Read the model definition and answer for the solid it produces. Units are mm, in the model's axes. Face numbers are marked on the shaded views. A direction names the side the tool comes from. Coordinates: 2 decimals unless noted, no trailing zeros. Loops run counter-clockwise (first coordinate to the right, second up) from the corner with the lowest first, then second, coordinate; pieces in that order, holes last. Notation, with made-up numbers: (59, 72) -> (111, 72) arc R20 ccw to (111, 105) -> close; hole circle Ø1 at (23, -21.75). An arc over 180 degrees is marked (long way). Answer as a JSON object with one key per item and string values. Group by question number.
1) Section B-B, the plane y = -0.5 is taken. Give the vertices of the cut face in (x, z), plus the area to 3 significant figures.
2) Which of the six approach directions +Z, -Z, +X, -X, +Y, -Y give full straight-line access (tool end or side, diameter ignored) to the marked faces 5 and 6?
3) Section C-C, the plane y = -6.5 is taken. Count the separate pieces of the cut face and the enclosed holes in it, plus the area to 3 significant figures.
4) Consider probe 1 along X at (y, z) = (-4, 12.25); probe 2 along Z at (x, y) = (45.5, -9.5); probe 3 along X at (y, z) = (2.5, 14.75). Determine where each line is inside the solid, lowest interval first. Write a range as [from, to].
5) Section D-D, the plane x = 41.5 is taken. Give the vertices of the cut face in (y, z), plus the area to 3 significant figures.
6) Section A-A, the plane x = 4.5 is taken. Give the vertices of the cut face in (y, z), plus the area to 3 significant figures.
7) Determine the mould class of the marked faces 1, 2, 3 and 4 for opening direction X: released by +X, released by -X, zero draft, split by the parting line, or undercut.
8) Flat-ended cylindrical pins translate along their axes: P1, Ø5, axis at x = 36.5, z = 13, coming from the +Y side; P2, Ø2, axis at x = 28, y = -6.5, coming from the -Z side. Find the tip coordinate at first contact, or state that the pin passes through.
from build123d import *

# Parameters (mm, degrees)
PRISM004_DEPTH            = 3
CYLINDER006_R             = 1.75
CYLINDER006_DEPTH         = 20
BOX006_W                  = 6
BOX006_H                  = 20
BOX006_DEPTH              = 3
FUSION004_PLACEMENT_ANGLE = 180
PRISM005_DEPTH            = 3
CYLINDER007_R             = 1.75
CYLINDER007_DEPTH         = 20
BOX007_W                  = 6
BOX007_H                  = 20
BOX007_DEPTH              = 3
FUSION005_PLACEMENT_ANGLE = 180
PRISM002_DEPTH            = 3
CYLINDER004_R             = 1.75
CYLINDER004_DEPTH         = 20
BOX003_W                  = 6
BOX003_H                  = 20
BOX003_DEPTH              = 3
FUSION001_PLACEMENT_ANGLE = 180
PRISM003_DEPTH            = 3
CYLINDER005_R             = 1.75
CYLINDER005_DEPTH         = 20
BOX005_W                  = 6
BOX005_H                  = 20
BOX005_DEPTH              = 3
FUSION002_PLACEMENT_ANGLE = 180
FUSION007_PLACEMENT_ANGLE = 180
PRISM006_DEPTH            = 3
CYLINDER008_R             = 1.75
CYLINDER008_DEPTH         = 20
BOX008_W                  = 6
BOX008_H                  = 20
BOX008_DEPTH              = 3
FUSION008_ROLL_ANGLE      = 90
FUSION008_PLACEMENT_ANGLE = 180
PRISM007_DEPTH            = 3
CYLINDER009_R             = 1.75
CYLINDER009_DEPTH         = 20
BOX009_W                  = 6
BOX009_H                  = 20
BOX009_DEPTH              = 3
FUSION009_ROLL_ANGLE      = 90
FUSION009_PLACEMENT_ANGLE = 180
CYLINDER001_R             = 1.5
CYLINDER001_DEPTH         = 10
CYLINDER_R                = 1.5
CYLINDER_DEPTH            = 10
BOX001_W                  = 46.6
BOX001_H                  = 10
BOX001_DEPTH              = 21
BOX_W                     = 49
BOX_H                     = 5
BOX_DEPTH                 = 15
BOX004_W                  = 49
BOX004_H                  = 16
BOX004_DEPTH              = 15


with BuildPart() as prisma004:
    # Prism004 → Prism004 (new body)
    with BuildSketch(Plane(origin=(34, 7.5, 3), x_dir=(0, 1, 0), z_dir=(0, 0, 1))):
        Polygon((3.25, 0), (1.625, 2.814583), (-1.625, 2.814583), (-3.25, 0), (-1.625, -2.814583), (1.625, -2.814583), align=None)
    extrude(amount=PRISM004_DEPTH)


with BuildPart() as cilindro006:
    # Cylinder006 → Cylinder006 (new body)
    with BuildSketch(Plane(origin=(34, 7.5, -1), x_dir=(1, 0, 0), z_dir=(0, 0, 1))):
        Circle(CYLINDER006_R)
    extrude(amount=CYLINDER006_DEPTH)


with BuildPart() as fusion004:
    # Box006 → Box006 (new body)
    with BuildSketch(Plane(origin=(31, 9, 3), x_dir=(1, 0, 0), z_dir=(0, 0, 1))):
        with Locations((3, 10)):
            Rectangle(BOX006_W, BOX006_H)
    extrude(amount=BOX006_DEPTH)

    # Fusion004: union Prisma004, Cilindro006
    add(prisma004.part)
    add(cilindro006.part)


with BuildPart() as fusion004_1:
    # Fusion004 placement: moved
    add(fusion004.part.moved(Location((-14, -3, 16))).rotate(Axis((-14, -3, 16), (1, 0, 0)), FUSION004_PLACEMENT_ANGLE))


with BuildPart() as prisma005:
    # Prism005 → Prism005 (new body)
    with BuildSketch(Plane(origin=(34, 7.5, 3), x_dir=(0, 1, 0), z_dir=(0, 0, 1))):
        Polygon((3.25, 0), (1.625, 2.814583), (-1.625, 2.814583), (-3.25, 0), (-1.625, -2.814583), (1.625, -2.814583), align=None)
    extrude(amount=PRISM005_DEPTH)


with BuildPart() as cilindro007:
    # Cylinder007 → Cylinder007 (new body)
    with BuildSketch(Plane(origin=(34, 7.5, -1), x_dir=(1, 0, 0), z_dir=(0, 0, 1))):
        Circle(CYLINDER007_R)
    extrude(amount=CYLINDER007_DEPTH)


with BuildPart() as fusion006:
    # Box007 → Box007 (new body)
    with BuildSketch(Plane(origin=(31, 9, 3), x_dir=(1, 0, 0), z_dir=(0, 0, 1))):
        with Locations((3, 10)):
            Rectangle(BOX007_W, BOX007_H)
    extrude(amount=BOX007_DEPTH)

    # Fusion005: union Prisma005, Cilindro007
    add(prisma005.part)
    add(cilindro007.part)


with BuildPart() as fusion006_1:
    # Fusion005 placement: moved
    add(fusion006.part.moved(Location((2, -3, 16))).rotate(Axis((2, -3, 16), (1, 0, 0)), FUSION005_PLACEMENT_ANGLE))

    # Fusion006: union Fusion004
    add(fusion004_1.part)


with BuildPart() as prisma002:
    # Prism002 → Prism002 (new body)
    with BuildSketch(Plane(origin=(34, 7.5, 3), x_dir=(0, 1, 0), z_dir=(0, 0, 1))):
        Polygon((3.25, 0), (1.625, 2.814583), (-1.625, 2.814583), (-3.25, 0), (-1.625, -2.814583), (1.625, -2.814583), align=None)
    extrude(amount=PRISM002_DEPTH)


with BuildPart() as cilindro004:
    # Cylinder004 → Cylinder004 (new body)
    with BuildSketch(Plane(origin=(34, 7.5, -1), x_dir=(1, 0, 0), z_dir=(0, 0, 1))):
        Circle(CYLINDER004_R)
    extrude(amount=CYLINDER004_DEPTH)


with BuildPart() as fusion001:
    # Box003 → Box003 (new body)
    with BuildSketch(Plane(origin=(31, 9, 3), x_dir=(1, 0, 0), z_dir=(0, 0, 1))):
        with Locations((3, 10)):
            Rectangle(BOX003_W, BOX003_H)
    extrude(amount=BOX003_DEPTH)

    # Fusion001: union Prisma002, Cilindro004
    add(prisma002.part)
    add(cilindro004.part)


with BuildPart() as fusion001_1:
    # Fusion001 placement: moved
    add(fusion001.part.moved(Location((47, -3, 0))).rotate(Axis((47, -3, 0), (0, 0, 1)), FUSION001_PLACEMENT_ANGLE))


with BuildPart() as prisma003:
    # Prism003 → Prism003 (new body)
    with BuildSketch(Plane(origin=(34, 7.5, 3), x_dir=(0, 1, 0), z_dir=(0, 0, 1))):
        Polygon((3.25, 0), (1.625, 2.814583), (-1.625, 2.814583), (-3.25, 0), (-1.625, -2.814583), (1.625, -2.814583), align=None)
    extrude(amount=PRISM003_DEPTH)


with BuildPart() as cilindro005:
    # Cylinder005 → Cylinder005 (new body)
    with BuildSketch(Plane(origin=(34, 7.5, -1), x_dir=(1, 0, 0), z_dir=(0, 0, 1))):
        Circle(CYLINDER005_R)
    extrude(amount=CYLINDER005_DEPTH)


with BuildPart() as fusion007:
    # Box005 → Box005 (new body)
    with BuildSketch(Plane(origin=(31, 9, 3), x_dir=(1, 0, 0), z_dir=(0, 0, 1))):
        with Locations((3, 10)):
            Rectangle(BOX005_W, BOX005_H)
    extrude(amount=BOX005_DEPTH)

    # Fusion002: union Prisma003, Cilindro005
    add(prisma003.part)
    add(cilindro005.part)


with BuildPart() as fusion007_1:
    # Fusion002 placement: moved
    add(fusion007.part.moved(Location((62, -3, 0))).rotate(Axis((62, -3, 0), (0, 0, 1)), FUSION002_PLACEMENT_ANGLE))

    # Fusion003: union Fusion001
    add(fusion001_1.part)

    # Fusion007: union Fusion006
    add(fusion006_1.part)


with BuildPart() as fusion007_2:
    # Fusion007 placement: moved
    add(fusion007_1.part.moved(Location((0, -17, 16))).rotate(Axis((0, -17, 16), (1, 0, 0)), FUSION007_PLACEMENT_ANGLE))


with BuildPart() as prisma006:
    # Prism006 → Prism006 (new body)
    with BuildSketch(Plane(origin=(34, 7.5, 3), x_dir=(0, 1, 0), z_dir=(0, 0, 1))):
        Polygon((3.25, 0), (1.625, 2.814583), (-1.625, 2.814583), (-3.25, 0), (-1.625, -2.814583), (1.625, -2.814583), align=None)
    extrude(amount=PRISM006_DEPTH)


with BuildPart() as cilindro008:
    # Cylinder008 → Cylinder008 (new body)
    with BuildSketch(Plane(origin=(34, 7.5, -1), x_dir=(1, 0, 0), z_dir=(0, 0, 1))):
        Circle(CYLINDER008_R)
    extrude(amount=CYLINDER008_DEPTH)


with BuildPart() as fusion008:
    # Box008 → Box008 (new body)
    with BuildSketch(Plane(origin=(31, 9, 3), x_dir=(1, 0, 0), z_dir=(0, 0, 1))):
        with Locations((3, 10)):
            Rectangle(BOX008_W, BOX008_H)
    extrude(amount=BOX008_DEPTH)

    # Fusion008: union Prisma006, Cilindro008
    add(prisma006.part)
    add(cilindro008.part)


with BuildPart() as fusion008_1:
    # Fusion008 roll: moved
    add(fusion008.part.rotate(Axis((0, 0, 0), (1, 0, 0)), FUSION008_ROLL_ANGLE))


with BuildPart() as fusion008_2:
    # Fusion008 placement: moved
    add(fusion008_1.part.moved(Location((37.5, -11, -4))).rotate(Axis((37.5, -11, -4), (0, 0, 1)), FUSION008_PLACEMENT_ANGLE))


with BuildPart() as prisma007:
    # Prism007 → Prism007 (new body)
    with BuildSketch(Plane(origin=(34, 7.5, 3), x_dir=(0, 1, 0), z_dir=(0, 0, 1))):
        Polygon((3.25, 0), (1.625, 2.814583), (-1.625, 2.814583), (-3.25, 0), (-1.625, -2.814583), (1.625, -2.814583), align=None)
    extrude(amount=PRISM007_DEPTH)


with BuildPart() as cilindro009:
    # Cylinder009 → Cylinder009 (new body)
    with BuildSketch(Plane(origin=(34, 7.5, -1), x_dir=(1, 0, 0), z_dir=(0, 0, 1))):
        Circle(CYLINDER009_R)
    extrude(amount=CYLINDER009_DEPTH)


with BuildPart() as fusion011:
    # Box009 → Box009 (new body)
    with BuildSketch(Plane(origin=(31, 9, 3), x_dir=(1, 0, 0), z_dir=(0, 0, 1))):
        with Locations((3, 10)):
            Rectangle(BOX009_W, BOX009_H)
    extrude(amount=BOX009_DEPTH)

    # Fusion009: union Prisma007, Cilindro009
    add(prisma007.part)
    add(cilindro009.part)


with BuildPart() as fusion011_1:
    # Fusion009 roll: moved
    add(fusion011.part.rotate(Axis((0, 0, 0), (1, 0, 0)), FUSION009_ROLL_ANGLE))


with BuildPart() as fusion011_2:
    # Fusion009 placement: moved
    add(fusion011_1.part.moved(Location((79.5, -11, -4))).rotate(Axis((79.5, -11, -4), (0, 0, 1)), FUSION009_PLACEMENT_ANGLE))

    # Fusion011: union Fusion007, Fusion008
    add(fusion007_2.part)
    add(fusion008_2.part)


with BuildPart() as cilindro001:
    # Cylinder001 → Cylinder001 (new body)
    with BuildSketch(Plane(origin=(45.7, 8, 3.2), x_dir=(1, 0, 0), z_dir=(0, -1, 0))):
        Circle(CYLINDER001_R)
    extrude(amount=CYLINDER001_DEPTH)


with BuildPart() as fusion:
    # Cylinder → Cylinder (new body)
    with BuildSketch(Plane(origin=(3.2, 8, 3.2), x_dir=(1, 0, 0), z_dir=(0, -1, 0))):
        Circle(CYLINDER_R)
    extrude(amount=CYLINDER_DEPTH)

    # Fusion: union Cilindro001
    add(cilindro001.part)


with BuildPart() as cubo001:
    # Box001 → Box001 (new body)
    with BuildSketch(Plane(origin=(1.2, 1.5, 1.2), x_dir=(1, 0, 0), z_dir=(0, 0, 1))):
        with Locations((23.3, 5)):
            Rectangle(BOX001_W, BOX001_H)
    extrude(amount=BOX001_DEPTH)


with BuildPart() as cut001:
    # Box → Box (new body)
    with BuildSketch(Plane.XY):
        with Locations((24.5, 2.5)):
            Rectangle(BOX_W, BOX_H)
    extrude(amount=BOX_DEPTH)

    # Cut: cut Cubo001
    add(cubo001.part, mode=Mode.SUBTRACT)

    # Cut001: cut Fusion
    add(fusion.part, mode=Mode.SUBTRACT)


with BuildPart() as cut002:
    # Box004 → Box004 (new body)
    with BuildSketch(Plane(origin=(0, -15, 0), x_dir=(1, 0, 0), z_dir=(0, 0, 1))):
        with Locations((24.5, 8)):
            Rectangle(BOX004_W, BOX004_H)
    extrude(amount=BOX004_DEPTH)

    # Fusion010: union Cut001
    add(cut001.part)

    # Cut002: cut Fusion011
    add(fusion011_2.part, mode=Mode.SUBTRACT)


solid = cut002.part
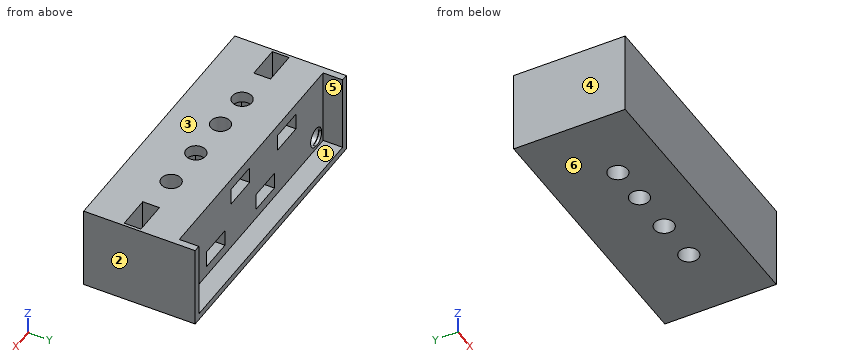
Determined:
{
 "1": {"outline": "(0, 0) -> (49, 0) -> (49, 15) -> (0, 15) -> close; hole circle Ø3.5 at (3.5, 3.5); hole (10, 10) -> (16, 10) -> (16, 13) -> (10, 13) -> close; hole (17, 3) -> (23, 3) -> (23, 6) -> (17, 6) -> close; hole (25, 10) -> (31, 10) -> (31, 13) -> (25, 13) -> close; hole (33, 3) -> (39, 3) -> (39, 6) -> (33, 6) -> close; hole circle Ø3.5 at (45.5, 3.5)", "area": "644 mm²"},
 "2": {"face 5": "+Z, +Y", "face 6": "-Z, +X, -X, +Y, -Y"},
 "3": {"separate pieces": "5", "enclosed holes": "0", "area": "335 mm²"},
 "4": {"probe 1": "[0, 10], [16, 25], [31, 49]", "probe 2": "[0, 1.75], [5.25, 15]", "probe 3": "[0, 1.2], [47.8, 49]"},
 "5": {"outline": "(-15, 0) -> (5, 0) -> (5, 1.2) -> (1.5, 1.2) -> (1.5, 15) -> (-15, 15) -> close", "area": "252 mm²"},
 "6": {"outline": "(-15, 0) -> (5, 0) -> (5, 1.2) -> (1.5, 1.2) -> (1.5, 2.06) -> (-5, 2.06) -> (-5, 0.83) -> (-8, 0.83) -> (-8, 2.06) -> (-12, 2.06) -> (-12, 4.94) -> (-8, 4.94) -> (-8, 15) -> (-15, 15) -> close; (-5, 4.94) -> (1.5, 4.94) -> (1.5, 15) -> (-5, 15) -> close", "area": "179 mm²"},
 "7": {"face 1": "undercut", "face 2": "released by +X", "face 3": "zero draft", "face 4": "released by -X"},
 "8": {"P1": "y = 1.5", "P2": "through"}
}
